Work out the finished part from the listing and answer in its coordinate system (mm). A direction names the side the tool comes from. Give positions to 0.01 mm unless a question says otherwise; leave off trailing zeros. Loops run counter-clockwise (first coordinate to the right, second up) from the corner with the lowest first, then second, coordinate; pieces in that order, holes last. Notation, with made-up numbers: M -40,78 L 0,78 A18 ccw 0,85 Z; hole C 76.25,64.25 d4. An arc over 180 degrees is marked long. Write item = value, one per line. Start each with the question number.
1. Consider L1, parallel to Z at x = 165.75, y = 7; L2, parallel to Y at x = 168, z = 101.5; L3, parallel to X at y = 38.5, z = 44. Determine where each line is inside the solid, lowest interval first. Write a range as [from, to].
2. Section B-B on z = 46 is taken. Determine the outline of the cut face in (x, y), plus the area to 4 significant figures.
3. Section D-D on z = 64 is taken. Determine the outline of the cut face in (x, y), plus the area to 3 significant figures.
4. The mould has two halves that part along Z. Classify faces 6 (the face through (164.771, 29.431, 52.164)), 7 (the face through (174.32, 11.73, 79.65)), 8 (the face through (165.7, 31.3, 120.3)), 9 (the face through (153.865, 29, 72)): released by +Z, released by -Z, zero draft, split by the parting line, or undercut.
5. Section C-C on x = 168 is taken. Determine the outline of the cut face in (y, z), plus the area to 3 significant figures.
6. Flat-ended cylindrical pins translate along their axes: pin 1 Ø5 at (y, z) = (11.6, 76.58) entering from -X; pin 2 Ø2 at (x, y) = (160.5, 2) entering from -Z; pin 3 Ø1.5 at (x, y) = (166, -4) entering from +Z; pin 4 Ø5 at (x, z) = (163.37, 49.68) entering from +Y. Find the tip coordinate at first contact, or state that the pin passes through.
7. For faces 1 (the face through (169.884, 30.982, 106.7)), 2 (the face through (167.91, 11.87, 82.68)), 3 (the face through (163, 39, 118.677)), 4 (the face through (171.456, 9.576, 67.808)), 5 (the face through (163, 26.749, 50)), determine the directions among +Z, -Z, +X, -X, +Y, -Y from which every point of the face is accessible in a straight line to the end or side of a thin tool.
8. Section A-A on z = 77 is taken. Determine the outline of the cut face in (x, y), plus the area to 3 significant figures.
```python
from build123d import *

# Parameters (mm, degrees)
SKETCH1_R           = 22.45
SKETCH1_R_2         = 6.11
SKETCH1_R_3         = 18.55
SKETCH1_R_4         = 5.25
SKETCH1_R_5         = 3.075
BOSS_EXTRUDE1_DEPTH = 5.5
SKETCH1_3_R         = 22.45
SKETCH1_3_R_2       = 6.11
SKETCH1_3_R_3       = 18.55
BOSS_EXTRUDE2_DEPTH = 6
BOSS_EXTRUDE3_START = -17
SKETCH1_4_R         = 18.55
BOSS_EXTRUDE3_DEPTH = 11
BOSS_EXTRUDE4_DEPTH = 10
DRAFT1_ANGLE        = 45
BOSS_EXTRUDE5_DEPTH = 3
SKETCH4_R           = 3.075
BOSS_EXTRUDE6_DEPTH = 1.5
CUT_EXTRUDE1_START  = -11
SKETCH3_4_R         = 1.55
CUT_EXTRUDE1_DEPTH  = 11
CUT_EXTRUDE2_START  = -9.6
SKETCH3_5_R         = 1.55
CUT_EXTRUDE2_DEPTH  = 2.6
CUT_EXTRUDE3_START  = -8
SKETCH3_6_R         = 1.55
CUT_EXTRUDE3_DEPTH  = 2.5
CUT_EXTRUDE4_DEPTH  = 13


with BuildPart() as part:
    # Sketch1 → Boss-Extrude1 (new body)
    with BuildSketch(Plane(origin=(170.865454796, 0, 0), x_dir=(0, 0, -1), z_dir=(1, 0, 0))):
        with BuildLine():
            ThreePointArc((-69.739907234, -12.350878767), (-85.614454471, -5.775426005), (-92.189907234, 10.099121233))
            Line((-92.189907234, 10.099121233), (-92.189907234, -12.350878767))
            Line((-92.189907234, -12.350878767), (-69.739907234, -12.350878767))
        make_face()
        with BuildLine():
            Line((-116.677399291, 29.749121233), (-92.189907234, 29.749121233))
            Line((-92.189907234, 29.749121233), (-92.189907234, 10.099121233))
            ThreePointArc((-92.189907234, 10.099121233), (-69.739907234, 32.549121233), (-47.289907234, 10.099121233))
            Line((-47.289907234, 10.099121233), (-47.289907234, 32.249121233))
            Line((-47.289907234, 32.249121233), (-41.977399291, 32.249121233))
            ThreePointArc((-41.977399291, 32.249121233), (-40.209632338, 32.98135428), (-39.477399291, 34.749121233))
            Line((-39.477399291, 34.749121233), (-39.477399291, 40.749121233))
            Line((-39.477399291, 40.749121233), (-42.477399291, 40.749121233))
            Line((-42.477399291, 40.749121233), (-42.477399291, 37.749121233))
            Line((-42.477399291, 37.749121233), (-118.677399291, 37.749121233))
            Line((-118.677399291, 37.749121233), (-118.677399291, 40.749121233))
            Line((-118.677399291, 40.749121233), (-121.677399291, 40.749121233))
            Line((-121.677399291, 40.749121233), (-121.677399291, 34.749121233))
            ThreePointArc((-121.677399291, 34.749121233), (-120.212933197, 31.213587327), (-116.677399291, 29.749121233))
        make_face()
        with BuildLine():
            Line((-47.289907234, -12.350878767), (-47.289907234, 10.099121233))
            ThreePointArc((-47.289907234, 10.099121233), (-53.865359996, -5.775426005), (-69.739907234, -12.350878767))
            Line((-69.739907234, -12.350878767), (-47.289907234, -12.350878767))
        make_face()
        with Locations((-69.739907234, 10.099121233)):
            Circle(SKETCH1_R)
        with Locations((-76.577399291, 11.598688626)):
            Circle(SKETCH1_R_2, mode=Mode.SUBTRACT)
        with Locations((-69.739907234, 10.099121233)):
            Circle(SKETCH1_R_3)
        with Locations((-76.577399291, 11.598688626)):
            Circle(SKETCH1_R_2, mode=Mode.SUBTRACT)
        with Locations((-76.577399291, 11.598688626)):
            Circle(SKETCH1_R_2)
        with Locations((-76.577399291, 11.598688626)):
            Circle(SKETCH1_R_4, mode=Mode.SUBTRACT)
        with Locations((-76.577399291, 11.598688626)):
            Circle(SKETCH1_R_4)
        with Locations((-76.577399291, 11.598688626)):
            Circle(SKETCH1_R_5, mode=Mode.SUBTRACT)
    extrude(amount=BOSS_EXTRUDE1_DEPTH)

    # Sketch1<3> → Boss-Extrude2 (add)
    with BuildSketch(Plane(origin=(170.865454796, 0, 0), x_dir=(0, 0, -1), z_dir=(1, 0, 0))):
        with BuildLine():
            ThreePointArc((-69.739907234, -12.350878767), (-85.614454471, -5.775426005), (-92.189907234, 10.099121233))
            Line((-92.189907234, 10.099121233), (-92.189907234, -12.350878767))
            Line((-92.189907234, -12.350878767), (-69.739907234, -12.350878767))
        make_face()
        with BuildLine():
            Line((-47.289907234, -12.350878767), (-47.289907234, 10.099121233))
            ThreePointArc((-47.289907234, 10.099121233), (-53.865359996, -5.775426005), (-69.739907234, -12.350878767))
            Line((-69.739907234, -12.350878767), (-47.289907234, -12.350878767))
        make_face()
        with BuildLine():
            Line((-116.677399291, 29.749121233), (-92.189907234, 29.749121233))
            Line((-92.189907234, 29.749121233), (-92.189907234, 10.099121233))
            ThreePointArc((-92.189907234, 10.099121233), (-69.739907234, 32.549121233), (-47.289907234, 10.099121233))
            Line((-47.289907234, 10.099121233), (-47.289907234, 32.249121233))
            Line((-47.289907234, 32.249121233), (-41.977399291, 32.249121233))
            ThreePointArc((-41.977399291, 32.249121233), (-40.209632338, 32.98135428), (-39.477399291, 34.749121233))
            Line((-39.477399291, 34.749121233), (-39.477399291, 40.749121233))
            Line((-39.477399291, 40.749121233), (-42.477399291, 40.749121233))
            Line((-42.477399291, 40.749121233), (-42.477399291, 37.749121233))
            Line((-42.477399291, 37.749121233), (-118.677399291, 37.749121233))
            Line((-118.677399291, 37.749121233), (-118.677399291, 40.749121233))
            Line((-118.677399291, 40.749121233), (-121.677399291, 40.749121233))
            Line((-121.677399291, 40.749121233), (-121.677399291, 34.749121233))
            ThreePointArc((-121.677399291, 34.749121233), (-120.212933197, 31.213587327), (-116.677399291, 29.749121233))
        make_face()
        with Locations((-69.739907234, 10.099121233)):
            Circle(SKETCH1_3_R)
        with Locations((-76.577399291, 11.598688626)):
            Circle(SKETCH1_3_R_2, mode=Mode.SUBTRACT)
        with Locations((-69.739907234, 10.099121233)):
            Circle(SKETCH1_3_R_3)
        with Locations((-76.577399291, 11.598688626)):
            Circle(SKETCH1_3_R_2, mode=Mode.SUBTRACT)
    extrude(amount=-BOSS_EXTRUDE2_DEPTH)

    # Sketch1<4> → Boss-Extrude3 (add)
    with BuildSketch(Plane(origin=(170.865454796, 0, 0), x_dir=(0, 0, -1), z_dir=(1, 0, 0)).offset(BOSS_EXTRUDE3_START)):
        with BuildLine():
            Line((-116.677399291, 29.749121233), (-92.189907234, 29.749121233))
            Line((-92.189907234, 29.749121233), (-92.189907234, -12.350878767))
            Line((-92.189907234, -12.350878767), (-47.289907234, -12.350878767))
            Line((-47.289907234, -12.350878767), (-47.289907234, 32.249121233))
            Line((-47.289907234, 32.249121233), (-41.977399291, 32.249121233))
            ThreePointArc((-41.977399291, 32.249121233), (-40.209632338, 32.98135428), (-39.477399291, 34.749121233))
            Line((-39.477399291, 34.749121233), (-39.477399291, 40.749121233))
            Line((-39.477399291, 40.749121233), (-42.477399291, 40.749121233))
            Line((-42.477399291, 40.749121233), (-42.477399291, 37.749121233))
            Line((-42.477399291, 37.749121233), (-118.677399291, 37.749121233))
            Line((-118.677399291, 37.749121233), (-118.677399291, 40.749121233))
            Line((-118.677399291, 40.749121233), (-121.677399291, 40.749121233))
            Line((-121.677399291, 40.749121233), (-121.677399291, 34.749121233))
            ThreePointArc((-121.677399291, 34.749121233), (-120.212933197, 31.213587327), (-116.677399291, 29.749121233))
        make_face()
        with Locations((-69.739907234, 10.099121233)):
            Circle(SKETCH1_4_R, mode=Mode.SUBTRACT)
    extrude(amount=BOSS_EXTRUDE3_DEPTH)

    # Sketch2 → Boss-Extrude4 (add)
    with BuildSketch(Plane.ZY.offset(-153.865454796)):
        with BuildLine():
            Line((56.448939974, 37.749121233), (96.705858608, 37.749121233))
            ThreePointArc((96.705858608, 37.749121233), (76.577399291, 44.598688626), (56.448939974, 37.749121233))
        make_face()
    extrude(amount=-BOSS_EXTRUDE4_DEPTH)

    # Draft1
    draft1_faces = [part.faces().sort_by_distance(p)[0] for p in [
        (163.865454796, 40.514883149, 76.577399291),
    ]]
    draft(draft1_faces, Plane(origin=(274.224792623, 37.749121233, 0), x_dir=(1, 0, 0), z_dir=(0, 1, 0)), DRAFT1_ANGLE)

    # Sketch3 → Boss-Extrude5 (add)
    with BuildSketch(Plane(origin=(0, 37.749121233, 0), x_dir=(1, 0, 0), z_dir=(0, 1, 0))):
        with BuildLine():
            Line((176.365454796, -118.677399291), (176.365454796, -115.477399292))
            ThreePointArc((176.365454796, -115.477399292), (174.926704491, -117.77896141), (172.365454796, -118.677399291))
            Line((172.365454796, -118.677399291), (176.365454796, -118.677399291))
        make_face()
    extrude(amount=BOSS_EXTRUDE5_DEPTH)

    # Sketch4 → Boss-Extrude6 (add)
    with BuildSketch(Plane(origin=(176.365454796, 0, 0), x_dir=(0, 0, -1), z_dir=(1, 0, 0))):
        with BuildLine():
            Line((-115.477399292, 37.749121233), (-115.477399292, 40.749121233))
            Line((-115.477399292, 40.749121233), (-121.677399291, 40.749121233))
            Line((-121.677399291, 40.749121233), (-121.677399291, 34.749121233))
            ThreePointArc((-121.677399291, 34.749121233), (-120.212933197, 31.213587327), (-116.677399291, 29.749121233))
            Line((-116.677399291, 29.749121233), (-92.189907234, 29.749121233))
            Line((-92.189907234, 29.749121233), (-92.189907234, -12.350878767))
            Line((-92.189907234, -12.350878767), (-47.289907234, -12.350878767))
            Line((-47.289907234, -12.350878767), (-47.289907234, 32.249121233))
            Line((-47.289907234, 32.249121233), (-41.977399291, 32.249121233))
            ThreePointArc((-41.977399291, 32.249121233), (-40.209632338, 32.98135428), (-39.477399291, 34.749121233))
            Line((-39.477399291, 34.749121233), (-39.477399291, 40.749121233))
            Line((-39.477399291, 40.749121233), (-42.477399291, 40.749121233))
            Line((-42.477399291, 40.749121233), (-42.477399291, 37.749121233))
            Line((-42.477399291, 37.749121233), (-53.314663543, 37.749121233))
            Line((-53.314663543, 37.749121233), (-99.840135039, 37.749121233))
            Line((-99.840135039, 37.749121233), (-115.477399292, 37.749121233))
        make_face()
        with Locations((-76.577399291, 11.598688626)):
            Circle(SKETCH4_R, mode=Mode.SUBTRACT)
        with BuildLine():
            Line((-95.948828739, 40.749121233), (-115.477399292, 40.749121233))
            Line((-115.477399292, 40.749121233), (-115.477399292, 37.749121233))
            Line((-115.477399292, 37.749121233), (-99.840135039, 37.749121233))
            ThreePointArc((-99.840135039, 37.749121233), (-97.9471913, 39.31749072), (-95.948828739, 40.749121233))
        make_face()
        with BuildLine():
            ThreePointArc((-57.205969843, 40.749121233), (-55.207607282, 39.31749072), (-53.314663543, 37.749121233))
            Line((-53.314663543, 37.749121233), (-42.477399291, 37.749121233))
            Line((-42.477399291, 37.749121233), (-42.477399291, 40.749121233))
            Line((-42.477399291, 40.749121233), (-57.205969843, 40.749121233))
        make_face()
    extrude(amount=BOSS_EXTRUDE6_DEPTH)

    # Sketch3<4> → Cut-Extrude1 (cut)
    with BuildSketch(Plane(origin=(0, 37.749121233, 0), x_dir=(1, 0, 0), z_dir=(0, 1, 0)).offset(CUT_EXTRUDE1_START)):
        with Locations(Location((172.340454796, -108.144978953, 0), (0, 0, 180))):
            Circle(SKETCH3_4_R)
        with Locations(Location((163.365454796, -49.683845424, 0), (0, 0, 180))):
            Circle(SKETCH3_4_R)
    extrude(amount=CUT_EXTRUDE1_DEPTH, mode=Mode.SUBTRACT)

    # Sketch3<5> → Cut-Extrude2 (cut)
    with BuildSketch(Plane(origin=(0, 37.749121233, 0), x_dir=(1, 0, 0), z_dir=(0, 1, 0)).offset(CUT_EXTRUDE2_START)):
        Polygon((164.91903222, -47.289907234), (161.811877372, -47.289907234), (160.515454796, -48.038397157), (160.515454796, -51.329293692), (163.365454796, -52.974741959), (166.215454796, -51.329293692), (166.215454796, -48.038397157), align=None)
        with Locations(Location((163.365454796, -49.683845424, 0), (0, 0, 180))):
            Circle(SKETCH3_5_R, mode=Mode.SUBTRACT)
        Polygon((166.215454796, -47.289907234), (164.91903222, -47.289907234), (166.215454796, -48.038397157), align=None)
        Polygon((160.515454796, -48.038397157), (161.811877372, -47.289907234), (160.515454796, -47.289907234), align=None)
    extrude(amount=CUT_EXTRUDE2_DEPTH, mode=Mode.SUBTRACT)

    # Sketch3<6> → Cut-Extrude3 (cut)
    with BuildSketch(Plane(origin=(0, 37.749121233, 0), x_dir=(1, 0, 0), z_dir=(0, 1, 0)).offset(CUT_EXTRUDE3_START)):
        Polygon((170.695006529, -110.994978953), (173.985903063, -110.994978953), (175.63135133, -108.144978953), (173.985903063, -105.294978953), (170.695006529, -105.294978953), (169.049558261, -108.144978953), align=None)
        with Locations(Location((172.340454796, -108.144978953, 0), (0, 0, 180))):
            Circle(SKETCH3_6_R, mode=Mode.SUBTRACT)
    extrude(amount=CUT_EXTRUDE3_DEPTH, mode=Mode.SUBTRACT)

    # Sketch5 → Cut-Extrude4 (cut)
    with BuildSketch(Plane(origin=(177.865454796, 0, 0), x_dir=(0, 0, -1), z_dir=(1, 0, 0))):
        with BuildLine():
            ThreePointArc((-65.174281564, 20.653980883), (-58.506884568, 7.635546229), (-70.01055365, -1.397693566))
            ThreePointArc((-70.01055365, -1.397693566), (-72.822049276, 0.768705961), (-71.5993125, 4.100778791))
            ThreePointArc((-71.5993125, 4.100778791), (-67.786338075, 9.670673406), (-68.918335583, 16.325076583))
            ThreePointArc((-68.918335583, 16.325076583), (-68.634368389, 19.863036052), (-65.174281564, 20.653980883))
        make_face()
    extrude(amount=-CUT_EXTRUDE4_DEPTH, mode=Mode.SUBTRACT)


solid = part.part
```
Verdict:
q1.L1 = [47.29, 58.67], [68.84, 72.55], [80.6, 92.19]
q1.L2 = [29.75, 37.75]
q1.L3 = [176.37, 177.87]
q2.outline = M 153.87,32.25 L 177.87,32.25 L 177.87,40.75 L 176.37,40.75 L 176.37,37.75 L 153.87,37.75 Z
q2.area = 136.5 mm2
q3.outline = M 153.87,-12.35 L 177.87,-12.35 L 177.87,0.13 L 164.87,0.13 L 164.87,-7.54 L 153.87,-7.54 Z; M 153.87,27.74 L 164.87,27.74 L 164.87,20.06 L 177.87,20.06 L 177.87,37.75 L 163.87,37.75 L 159.51,42.11 L 153.87,42.11 Z
q3.area = 589 mm2
q4.face_6 = released by -Z
q4.face_7 = undercut
q4.face_8 = released by +Z
q4.face_9 = zero draft
q5.outline = M -12.35,47.29 L 32.25,47.29 L 32.25,41.98 A2.5 ccw 34.75,39.48 L 40.75,39.48 L 40.75,42.48 L 37.75,42.48 L 37.75,118.68 L 40.75,118.68 L 40.75,121.68 L 34.75,121.68 A5 ccw 29.75,116.68 L 29.75,92.19 L -12.35,92.19 Z; hole M -1.4,70.01 A11.5 ccw 20.65,65.17 A3 ccw 16.33,68.92 A9 cw 4.1,71.6 A3 ccw Z; hole C 11.6,76.58 d12.22
q5.area = 2,220 mm2
q6.pin_1 = through
q6.pin_2 = 47.29
q6.pin_3 = 92.19
q6.pin_4 = 37.75
q7.face_1 = -Y
q7.face_2 = -X
q7.face_3 = -X, +Y
q7.face_4 = +X, -X
q7.face_5 = +Y
q8.outline = M 153.87,-12.35 L 177.87,-12.35 L 177.87,8.55 L 170.87,8.55 L 170.87,5.5 L 164.87,5.5 L 164.87,-6.97 L 153.87,-6.97 Z; M 153.87,27.17 L 164.87,27.17 L 164.87,17.69 L 170.87,17.69 L 170.87,14.64 L 177.87,14.64 L 177.87,37.75 L 163.87,37.75 L 157.02,44.6 L 153.87,44.6 Z
q8.area = 756 mm2
